Work out the finished part from the listing and answer in its coordinate system (mm). Face numbers are marked on the shaded views. Coordinates: 2 decimals unless noted, no trailing zeros. Loops run counter-clockwise (first coordinate to the right, second up) from the corner with the lowest first, then second, coordinate; pieces in that order, holes last. Notation, with made-up numbers: (38.5, 31.5) -> (54.5, 31.5) arc R17 cw to (54.5, 44.5) -> close; hole circle Ø2 at (37.25, -15). An arc over 180 degrees is marked (long way). Use a Markdown table: item, result. Add a question column.
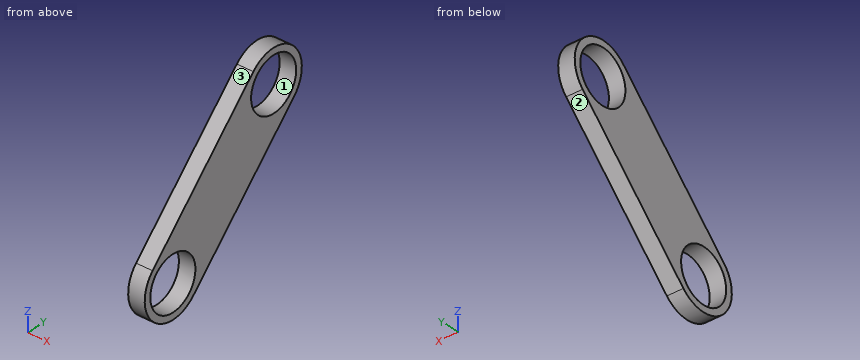
```python
from build123d import *

# Parameters (mm, degrees)
BOSS_EXTRUDE1_START = -4
SKETCH2_R           = 8
BOSS_EXTRUDE1_DEPTH = 5


with BuildPart() as part:
    # Sketch2 → Boss-Extrude1 (new body)
    with BuildSketch(Plane(origin=(0, 0, 0), x_dir=(0, 0, -1), z_dir=(1, 0, 0)).offset(BOSS_EXTRUDE1_START)):
        with BuildLine():
            Line((43.989770311, -28.585837543), (6.947291622, 7.192714309))
            ThreePointArc((6.947291622, 7.192714309), (-7.192714309, 6.947291622), (-6.947291622, -7.192714309))
            Line((-6.947291622, -7.192714309), (30.095187067, -42.97126616))
            ThreePointArc((30.095187067, -42.97126616), (44.235192998, -42.725843473), (43.989770311, -28.585837543))
        make_face()
        with Locations((37.042478689, -35.778551851)):
            Circle(SKETCH2_R, mode=Mode.SUBTRACT)
        Circle(SKETCH2_R, mode=Mode.SUBTRACT)
    extrude(amount=-BOSS_EXTRUDE1_DEPTH)


solid = part.part
```
Item 1: Find the intervals of material crossed by probe 1 along Z at (x, y) = (-4.85, -4); probe 2 along Z at (x, y) = (-6.7, -39); probe 3 along Y at (x, z) = (-8.55, -34.5), in increasing order.
Item 2: Given pin 1 (2 mm diameter, centred on x = -6.5, y = -2, fed in from +Z), flat-ended and moving along its own axis, determine where the tip first touches the part or whether it passes through.
Item 3: Section D-D (z = -10) is taken. Determine the outline of the cut face in (x, y).
Item 4: Section B-B (y = 0) is taken. Determine the outline of the cut face in (x, z), then the cut area to 3 significant figures.
Item 5: Section A-A (z = -31) is taken. Determine the outline of the cut face in (x, y), then the cut area to 3 significant figures.
Item 6: For a pull along Z with two mould halves and no side action, classify the marked faces 1, 2 and 3 as +Z half, -Z half, draft (parallel to the pull), parting line (faces both ways), or undercut.
Output:
| question | item | result |
|---|---|---|
| 1 | probe 1 | z = -18.54 to -6.93, 6.93 to 9.17 |
| 1 | probe 2 | z = -46.51 to -44.37, -29.72 to -25.98 |
| 1 | probe 3 | y = -45.45 to -43.36, -28.19 to -19.42 |
| 2 | pin 1 | stops at z = 9.95 |
| 3 | outline | (-9, -23.56) -> (-4, -23.56) -> (-4, 4.24) -> (-9, 4.24) -> close |
| 4 | outline | (-9, -14.39) -> (-4, -14.39) -> (-4, -8) -> (-9, -8) -> close; (-9, 8) -> (-4, 8) -> (-4, 10) -> (-9, 10) -> close |
| 4 | area | 42.0 mm2 |
| 5 | outline | (-9, -43.75) -> (-4, -43.75) -> (-4, -41.02) -> (-9, -41.02) -> close; (-9, -30.54) -> (-4, -30.54) -> (-4, -16.04) -> (-9, -16.04) -> close |
| 5 | area | 86.1 mm2 |
| 6 | face 1 | undercut |
| 6 | face 2 | -Z half |
| 6 | face 3 | +Z half |
